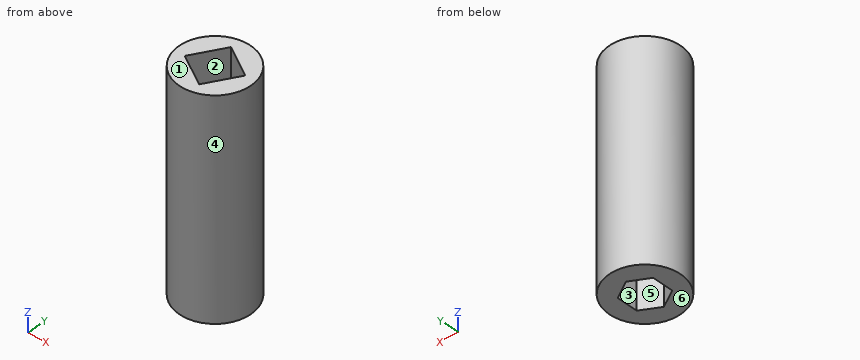
from build123d import *

# Parameters (mm, degrees)
SKETCH_R     = 10
PAD_DEPTH    = 50
SKETCH001_R  = 10
PAD001_DEPTH = 10


with BuildPart() as part:
    # Sketch → Pad (new body)
    with BuildSketch(Plane.XY):
        Circle(SKETCH_R)
        Polygon((5, -2.886751), (5, 2.886751), (0, 5.773503), (-5, 2.886751), (-5, -2.886751), (0, -5.773503), align=None, mode=Mode.SUBTRACT)
    extrude(amount=PAD_DEPTH)

    # Sketch001 → Pad001 (join)
    with BuildSketch(Plane.XY.offset(50)):
        Circle(SKETCH001_R)
        Polygon((-1.830127, 6.830127), (-6.830127, -1.830127), (1.830127, -6.830127), (6.830127, 1.830127), align=None, mode=Mode.SUBTRACT)
    extrude(amount=PAD001_DEPTH)


solid = part.part
Could you check a few things on this model? Use its own coordinates, in mm. Face numbers are marked on the shaded views. A direction names the side the tool comes from. Give positions to 0.01 mm unless a question says otherwise; leave off trailing zeros. Order: outer loops, then holes, each group sorted by start corner. A loop starts at its lowest first (then second) coordinate and runs counter-clockwise, first axis right, second up.
Item 1: If we section it at D-D, the plane y = -5: Write out the boundary of the cut face in (x, z), plus the area to 3 significant figures.
Item 2: If we section it at C-C, the plane x = -8: Write out the boundary of the cut face in (y, z), plus the area to 3 significant figures.
Item 3: If we section it at A-A, the plane y = 0: Write out the boundary of the cut face in (x, z).
Item 4: If we section it at B-B, the plane z = 42: Write out the boundary of the cut face in (x, y).
Item 5: I'm going to push flat-ended pins straight in: pin 1 (6 mm diameter, centred on x = 4.5, z = 22, fed in from -Y); pin 2 (6 mm diameter, centred on y = 7, z = 35.5, fed in from -X); pin 3 (8 mm diameter, centred on x = -8, z = 23, fed in from -Y). Where does each tip first touch, or does it pass through?
Item 6: I need wall thicknesses on line 1 (X direction, y = -1, z = 42); line 2 (X direction, y = -0.5, z = 3); line 3 (Y direction, x = 4.25, z = 10.5). Which ranges of each line are inside material? Lowest first, please.
Item 7: For the marked faces 1, 2 and 3, which set-ups out of +Z, -Z, +X, -X, +Y, -Y let a thin tool reach every point of the face, with its end or its side?
Item 8: If we mould it in two halves opening along Y, with no side actions, what happens to the marked faces 4, 5 and 6? For each: pulls with the +Y half, pulls with the -Y half, needs draft (parallel to the pull), parting line crosses it, or undercut.
Values:
1. outline: (-8.66, 0) - (-1.34, 0) - (-1.34, 60) - (-8.66, 60) - close; (1.34, 0) - (8.66, 0) - (8.66, 60) - (2.89, 60) - (2.89, 50) - (1.34, 50) - close
1. area: 863 mm2
2. outline: (-6, 0) - (6, 0) - (6, 60) - (-6, 60) - close
2. area: 720 mm2
3. outline: (-10, 0) - (-5, 0) - (-5, 50) - (-5.77, 50) - (-5.77, 60) - (-10, 60) - close; (5, 0) - (10, 0) - (10, 60) - (5.77, 60) - (5.77, 50) - (5, 50) - close
4. outline: circle Ø20 at (0, 0); hole (-5, -2.89) - (0, -5.77) - (5, -2.89) - (5, 2.89) - (0, 5.77) - (-5, 2.89) - close
5. pin 1: stops at y = -9.89
5. pin 2: stops at x = -9.17
5. pin 3: stops at y = -9.17
6. line 1: x = -9.95 to -5, 5 to 9.95
6. line 2: x = -9.99 to -5, 5 to 9.99
6. line 3: y = -9.05 to -3.32, 3.32 to 9.05
7. face 1: +Z, +X, -X, +Y, -Y
7. face 2: +Z
7. face 3: -Z
8. face 4: parting line crosses it
8. face 5: undercut
8. face 6: needs draft
